For this review, take the finished solid that the model builds, in its own axes (mm). A direction names the side the tool comes from. Coordinates: 2 decimals unless noted, no trailing zeros. Loops run counter-clockwise (first coordinate to the right, second up) from the corner with the lowest first, then second, coordinate; pieces in that order, holes last. Notation, with made-up numbers: (-32, -17) - (7, -17) arc R3 ccw to (7, -13) - close; hole circle Ø7 at (37.25, -6). An arc over 180 degrees is marked (long way). Answer as a JSON object with one key per item and string values. Group by question number.
Item 1: We need section C-C (z = -3.5). Give the boundary of the cut face in (x, y).
Item 2: Tool access review of faces 4 (the cylindrical face through (-1.73, 7.81, -4.45)), 5 (the flat face through (-21, 0, -4)): name each direction out of +Z, -Z, +X, -X, +Y, -Y from which nothing blocks a thin tool from reaching the whole face with its end or side.
Item 3: Clearance check with flat-ended pins moving along their axes: pin 1 (15 mm diameter, centred on x = 0, y = 0, fed in from +Z); pin 2 (14.5 mm diameter, centred on x = 0, y = 0, fed in from -Z); pin 3 (1 mm diameter, centred on x = -5, z = 1, fed in from -Y). State where each tip first meets the part, or that it passes through.
Item 4: To check wall thickness, follow line 1 (Y direction, x = 0, z = -3.75); line 2 (Y direction, x = 0, z = 0.2); line 3 (Z direction, x = -13.5, y = -10). State the ranges of each line that lie inside material, in increasing order.
Item 5: We need section A-A (x = 0). Give the boundary of the cut face in (y, z), then the cut area to 3 significant figures.
Item 6: We need section B-B (y = -15.5). Give the boundary of the cut face in (x, z).
Item 7: Mouldability with a two-part tool opening along X and no side actions: class faces 1 (the flat face through (-19.1, -19.05, -4)), 2 (the flat face through (3.44, 3.44, -0.9)), 3 (the flat face through (5, -2, 2)) as released by +X, released by -X, zero draft, split by the parting line, or undercut.
from build123d import *

# Parameters (mm, degrees)
SKETCH_R          = 11
PAD_DEPTH         = 2
PAD001_DEPTH      = 7.9
SKETCH002_R       = 4.7
POCKET_DEPTH      = 7.901
POCKET_DEPTH_BACK = 2.001
SKETCH003_R       = 1.25
HOLE_DEPTH        = 7.901
SKETCH004_R       = 8
POCKET001_DEPTH   = 7
CHAMFER_SIZE      = 0.2


with BuildPart() as part:
    # Sketch → Pad (new body)
    with BuildSketch(Plane.XY):
        Circle(SKETCH_R)
    extrude(amount=PAD_DEPTH)

    # Sketch001 → Pad001 (join)
    with BuildSketch(Plane.XY):
        Polygon((-21, 17.15), (-21, -17.15), (-17.15, -21), (17.15, -21), (21, -17.15), (21, 17.15), (17.15, 21), (-17.15, 21), align=None)
    extrude(amount=-PAD001_DEPTH)

    # Sketch002 → Pocket (cut, two sides)
    with BuildSketch(Plane.XY) as pocket_sk:
        Circle(SKETCH002_R)
    extrude(amount=-POCKET_DEPTH, mode=Mode.SUBTRACT)
    extrude(pocket_sk.sketch, amount=POCKET_DEPTH_BACK, mode=Mode.SUBTRACT)

    # Sketch003 → Hole (cut, through all)
    with BuildSketch(Plane.XY):
        with Locations((-15.5, 15.5)):
            Circle(SKETCH003_R)
        with Locations((15.5, 15.5)):
            Circle(SKETCH003_R)
        with Locations((15.5, -15.5)):
            Circle(SKETCH003_R)
        with Locations((-15.5, -15.5)):
            Circle(SKETCH003_R)
    extrude(amount=-HOLE_DEPTH, mode=Mode.SUBTRACT)

    # Sketch004 → Pocket001 (cut)
    with BuildSketch(Plane(origin=(0, 0, -7.9), x_dir=(1, 0, 0), z_dir=(0, 0, -1))):
        Circle(SKETCH004_R)
    extrude(amount=-POCKET001_DEPTH, mode=Mode.SUBTRACT)

    # Chamfer
    chamfer_edges = [part.edges().sort_by_distance(p)[0] for p in [
        (-21, 0, 0),
        (-19.075, 19.075, 0),
        (-19.075, -19.075, 0),
        (0, 21, 0),
        (0, -21, 0),
        (19.075, 19.075, 0),
        (19.075, -19.075, 0),
        (21, 0, 0),
        (-16.75, -15.5, 0),
        (-16.75, 15.5, 0),
        (-11, 0, 0),
        (14.25, 15.5, 0),
        (14.25, -15.5, 0),
        (-11, 0, 2),
        (-4.7, 0, 2),
    ]]
    chamfer(chamfer_edges, length=CHAMFER_SIZE)


solid = part.part
Check sheet entries:
{
 "1": {"outline": "(-21, -17.15) - (-17.15, -21) - (17.15, -21) - (21, -17.15) - (21, 17.15) - (17.15, 21) - (-17.15, 21) - (-21, 17.15) - close; hole circle Ø2.5 at (-15.5, -15.5); hole circle Ø2.5 at (-15.5, 15.5); hole circle Ø16 at (0, 0); hole circle Ø2.5 at (15.5, -15.5); hole circle Ø2.5 at (15.5, 15.5)"},
 "2": {"face 4": "-Z", "face 5": "+Z, -Z, -X, +Y, -Y"},
 "3": {"pin 1": "stops at z = 2", "pin 2": "stops at z = -0.9", "pin 3": "stops at y = -10.04"},
 "4": {"line 1": "y = -21 to -8, 8 to 21", "line 2": "y = -11 to -4.7, 4.7 to 11", "line 3": "z = -7.9 to 0"},
 "5": {"outline": "(-21, -7.9) - (-8, -7.9) - (-8, -0.9) - (-4.7, -0.9) - (-4.7, 1.8) - (-4.9, 2) - (-10.8, 2) - (-11, 1.8) - (-11, 0.2) - (-11.2, 0) - (-20.8, 0) - (-21, -0.2) - close; (4.7, -0.9) - (8, -0.9) - (8, -7.9) - (21, -7.9) - (21, -0.2) - (20.8, 0) - (11.2, 0) - (11, 0.2) - (11, 1.8) - (10.8, 2) - (4.9, 2) - (4.7, 1.8) - close", "area": "236 mm2"},
 "6": {"outline": "(-21, -7.9) - (-16.75, -7.9) - (-16.75, -0.2) - (-16.95, 0) - (-20.8, 0) - (-21, -0.2) - close; (-14.25, -7.9) - (14.25, -7.9) - (14.25, -0.2) - (14.05, 0) - (-14.05, 0) - (-14.25, -0.2) - close; (16.75, -7.9) - (21, -7.9) - (21, -0.2) - (20.8, 0) - (16.95, 0) - (16.75, -0.2) - close"},
 "7": {"face 1": "released by -X", "face 2": "undercut", "face 3": "zero draft"}
}
